Check sheet for the modelled part. Datum: model origin and axes. Units: mm. Round coordinates to 2 decimals unless told otherwise and drop trailing zeros. Order: outer loops, then holes, each group sorted by start corner. A loop starts at its lowest first (then second) coordinate and runs counter-clockwise, first axis right, second up. Notation, with made-up numbers: M 39.5,64 L 94.5,64 A30 ccw 94.5,101 Z; hole C 43.25,-4.5 d2. An arc over 180 degrees is marked long. One line per item, written item: value. Start each with the question number.
(1) Cross-section at A-A, the plane y = -28. Enter the section's corners in (x, z).
(2) Cross-section at D-D, the plane x = -15. Enter the section's corners in (y, z), and give its area (3 significant figures).
(3) Cross-section at B-B, the plane x = -128.5. Enter the section's corners in (y, z), and give its area (3 significant figures).
(4) Thickness scan on L1, parallel to X at y = -5, z = 1.65; L2, parallel to Y at x = -128.5, z = 1.15; L3, parallel to Y at x = -111.5, z = 0.4. Record the ranges inside material, lowest first.
(5) Cross-section at C-C, the plane z = 0.6. Count the separate pieces of the cut face and the enclosed holes in it, and give its area (3 significant figures).
(6) Depth check by flat-ended pin: pin 1 Ø5 at (x, y) = (-71.5, 23.5) entering from -Z; pin 2 Ø1 at (y, z) = (-58.5, 1.5) entering from -X; pin 3 Ø0.6 at (y, z) = (-14.5, 1) entering from -X; pin 4 Ø0.6 at (x, z) = (-106, 0.5) entering from -Y. Enter the tip coordinate at first touch or a pass-through.
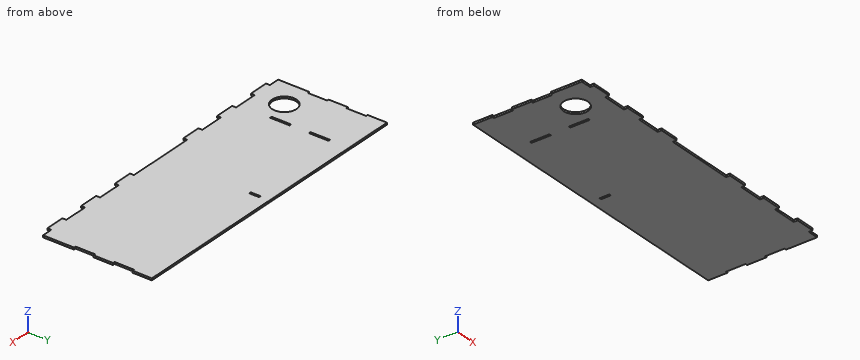
from build123d import *

# Parameters (mm, degrees)
SKETCH2_R               = 12.5
SKETCH2_W               = 2
SKETCH2_H               = 20
BOSS_EXTRUDE1_DEPTH     = 2
CUT_EXTRUDE1_DEPTH      = 168.619360457
CUT_EXTRUDE1_DEPTH_BACK = 168.619360457
SKETCH3_W               = 20
SKETCH3_H               = 2
CUT_EXTRUDE2_DEPTH      = 168.619360457
CUT_EXTRUDE2_DEPTH_BACK = 168.619360457
SKETCH5_W               = 2
SKETCH5_H               = 10


with BuildPart() as part:
    # Sketch2 → Boss-Extrude1 (new body)
    with BuildSketch(Plane.XY):
        Polygon((-100.5, -56), (-100.5, -60), (-80.5, -60), (-80.5, -56), (-55.5, -56), (-55.5, -60), (-35.5, -60), (-35.5, -56), (35.5, -56), (35.5, -60), (55.5, -60), (55.5, -56), (80.5, -56), (80.5, -60), (100.5, -60), (100.5, -56), (125.5, -56), (125.5, -60), (145.5, -60), (145.5, -56), (156.5, -56), (156.5, -24), (154.5, -24), (154.5, -4), (156.5, -4), (156.5, 16), (154.5, 16), (154.5, 36), (156.5, 36), (156.5, 56), (145.5, 56), (145.5, 58), (125.5, 58), (125.5, 56), (100.5, 56), (100.5, 58), (80.5, 58), (80.5, 56), (55.5, 56), (55.5, 58), (35.5, 58), (35.5, 56), (-35.5, 56), (-35.5, 58), (-55.5, 58), (-55.5, 56), (-80.5, 56), (-80.5, 58), (-100.5, 58), (-100.5, 56), (-125.5, 56), (-125.5, 58), (-145.5, 58), (-145.5, 56), (-156.5, 56), (-156.5, 36), (-154.5, 36), (-154.5, 16), (-156.5, 16), (-156.5, -4), (-154.5, -4), (-154.5, -24), (-156.5, -24), (-156.5, -56), (-145.5, -56), (-145.5, -60), (-125.5, -60), (-125.5, -56), align=None)
        with Locations((-128.5, -28)):
            Circle(SKETCH2_R, mode=Mode.SUBTRACT)
        with Locations((-105.5, 26)):
            Rectangle(SKETCH2_W, SKETCH2_H, mode=Mode.SUBTRACT)
        with Locations((-105.5, -14)):
            Rectangle(SKETCH2_W, SKETCH2_H, mode=Mode.SUBTRACT)
    extrude(amount=BOSS_EXTRUDE1_DEPTH)

    # Sketch3 → Cut-Extrude1 (cut, two sides: drawn at the far end of the back side and taken through both)
    with BuildSketch(Plane.XY.offset(2).offset(-CUT_EXTRUDE1_DEPTH_BACK)):
        with Locations((-135.5, 57)):
            Rectangle(SKETCH3_W, SKETCH3_H)
        with Locations((-90.5, 57)):
            Rectangle(SKETCH3_W, SKETCH3_H)
        with Locations((-45.5, 57)):
            Rectangle(SKETCH3_W, SKETCH3_H)
        with Locations((45.5, 57)):
            Rectangle(SKETCH3_W, SKETCH3_H)
        with Locations((90.5, 57)):
            Rectangle(SKETCH3_W, SKETCH3_H)
        with Locations((135.5, 57)):
            Rectangle(SKETCH3_W, SKETCH3_H)
    extrude(amount=CUT_EXTRUDE1_DEPTH + CUT_EXTRUDE1_DEPTH_BACK, mode=Mode.SUBTRACT)

    # Sketch5 → Cut-Extrude2 (cut, two sides: drawn at the far end of the back side and taken through both)
    with BuildSketch(Plane.XY.offset(2).offset(-CUT_EXTRUDE2_DEPTH_BACK)):
        with Locations((0, 41)):
            Rectangle(SKETCH5_W, SKETCH5_H)
    extrude(amount=CUT_EXTRUDE2_DEPTH + CUT_EXTRUDE2_DEPTH_BACK, mode=Mode.SUBTRACT)


solid = part.part
Values found:
1. outline: M -156.5,0 L -141,0 L -141,2 L -156.5,2 Z; M -116,0 L 156.5,0 L 156.5,2 L -116,2 Z
2. outline: M -56,0 L 56,0 L 56,2 L -56,2 Z
2. area: 224 mm^2
3. outline: M -60,0 L -40.5,0 L -40.5,2 L -60,2 Z; M -15.5,0 L 56,0 L 56,2 L -15.5,2 Z
3. area: 182 mm^2
4. L1: -154.5 to -106.5, -104.5 to 154.5
4. L2: -60 to -40.5, -15.5 to 56
4. L3: -56 to 56
5. separate pieces: 1
5. enclosed holes: 4
5. area: 34,800 mm^2
6. pin 1: z = 0
6. pin 2: x = -145.5
6. pin 3: x = -154.5
6. pin 4: y = -56
